from build123d import *

# Parameters (mm, degrees)
F1_DEPTH  = 15
F2_W      = 70
F2_H      = 100
F3_DEPTH  = 5
F4_W      = 40
F4_H      = 50
F5_DEPTH  = 25
F7_DEPTH  = 40
F9_DEPTH  = 40
F11_DEPTH = 3
F13_DEPTH = 1.5
F14_DEPTH = 1.5


with BuildPart() as f1:
    # F0 (on Front) → F1 (new body)
    with BuildSketch(Plane.XZ):
        with BuildLine():
            ThreePointArc((-80, 0), (-87.071068, -2.928932), (-90, -10))
            Line((-90, -10), (-90, -110))
            ThreePointArc((-90, -110), (-87.071068, -117.071068), (-80, -120))
            Line((-80, -120), (-10, -120))
            ThreePointArc((-10, -120), (-2.928932, -117.071068), (0, -110))
            Line((0, -110), (0, -10))
            ThreePointArc((0, -10), (-2.928932, -2.928932), (-10, 0))
            Line((-10, 0), (-80, 0))
        make_face()
    extrude(amount=F1_DEPTH)

    # F2 (on face) → F3 (cut)
    with BuildSketch(Plane.XZ.offset(15)):
        with Locations((-45, -60)):
            Rectangle(F2_W, F2_H)
    extrude(amount=-F3_DEPTH, mode=Mode.SUBTRACT)

    # F4 (on face) → F5 (join)
    with BuildSketch(Plane(origin=(0, 0, 0), x_dir=(-1, 0, 0), z_dir=(0, 1, 0))):
        with Locations((45, -25)):
            Rectangle(F4_W, F4_H)
    extrude(amount=F5_DEPTH)

    # F6 (on face) → F7 (cut)
    with BuildSketch(Plane(origin=(-65, 0, 0), x_dir=(0, -1, 0), z_dir=(-1, 0, 0))):
        Polygon((0, -39.708052), (0, 0), (-25, 0), align=None)
        Polygon((-25, -9.351011), (-25, -50), (0, -50), align=None)
    extrude(amount=-F7_DEPTH, mode=Mode.SUBTRACT)

    # F8 (on face) → F9 (cut)
    with BuildSketch(Plane(origin=(-65, 0, 0), x_dir=(0, -1, 0), z_dir=(-1, 0, 0))):
        with BuildLine():
            Line((-19.594347, -8.585918), (-25, 0))
            Line((-25, 0), (-25, -9.351011))
            Line((-25, -9.351011), (-24.627329, -8.520231))
            ThreePointArc((-24.627329, -8.520231), (-23.514035, -7.469649), (-21.983944, -7.513993))
            Line((-21.983944, -7.513993), (-19.594347, -8.585918))
        make_face()
    extrude(amount=-F9_DEPTH, mode=Mode.SUBTRACT)

    # F10 (on face) → F11 (join)
    with BuildSketch(Plane.XZ.offset(10)):
        Polygon((-20, -15), (-15, -20), (-15, -15), align=None)
        Polygon((-70, -105), (-75, -100), (-75, -105), align=None)
        Polygon((-75, -20), (-70, -15), (-75, -15), align=None)
        Polygon((-15, -100), (-20, -105), (-15, -105), align=None)
    extrude(amount=F11_DEPTH)

    # F12 (on face) → F13 (cut)
    with BuildSketch(Plane.XZ.offset(10)):
        Polygon((-74, -19), (-71, -16), (-74, -16), align=None)
        Polygon((-19, -16), (-16, -19), (-16, -16), align=None)
        Polygon((-71, -104), (-74, -101), (-74, -104), align=None)
        Polygon((-16, -101), (-19, -104), (-16, -104), align=None)
    extrude(amount=F13_DEPTH, mode=Mode.SUBTRACT)

    # F12 (on face) → F14 (cut)
    with BuildSketch(Plane.XZ.offset(10)):
        Polygon((-74, -19), (-71, -16), (-74, -16), align=None)
        Polygon((-19, -16), (-16, -19), (-16, -16), align=None)
        Polygon((-71, -104), (-74, -101), (-74, -104), align=None)
        Polygon((-16, -101), (-19, -104), (-16, -104), align=None)
    extrude(amount=F14_DEPTH, mode=Mode.SUBTRACT)


solid = f1.part
Work out the finished part from the listing and answer in its coordinate system (mm). A direction names the side the tool comes from. Coordinates: 2 decimals unless noted, no trailing zeros. Loops run counter-clockwise (first coordinate to the right, second up) from the corner with the lowest first, then second, coordinate; pieces in that order, holes last. Notation, with made-up numbers: (68.25, 35.25) -> (121.25, 35.25) arc R34 cw to (121.25, 74.25) -> close; hole circle Ø1 at (89, 14). An arc over 180 degrees is marked (long way). Write each question's results on one line, items separated by ' | '. Start each with the question number.
1) Consider line 1 along Z through (x, y) = (-26.5, -10.5); line 2 along X through (y, z) = (-12.5, -47); line 3 along Y through (x, z) = (-9, -56). Determine where each line is inside the solid, lowest interval first.
2) For faces 1 (the flat face through (-65, 11, -27)), 2 (the flat face through (-17, -11.5, -17)), 3 (the flat face through (-17, -12, -102)), 4 (the cylindrical face through (-86.99, -7.4, -2.85)), 5 (the cylindrical face through (-87.15, -7.4, -116.99)), determine the directions among +Z, -Z, +X, -X, +Y, -Y from which every point of the face is accessible in a straight line to the end or side of a thin tool.
3) Find section A-A on x = -23.5. Determine the outline of the cut face in (y, z).
4) The mould has two halves that part along Y. Classify faces 6 (the flat face through (-17, -11.5, -103)), 7 (the flat face through (-45.3, 12.3, -30)), 8 (the flat face through (-18, -12, -17)): pulls with the +Y half, pulls with the -Y half, needs draft (parallel to the pull), parting line crosses it, or undercut.
5) Find section C-C on z = -96.5. Determine the outline of the cut face in (x, y), then the cut area to 3 significant figures.
6) Find section D-D on x = -59. Determine the outline of the cut face in (y, z), then the cut area to 3 significant figures.
7) Flat-ended cylindrical pins translate along their axes: P1, Ø2.5, axis at x = -71.5, z = -16.5, coming from the -Y side; P2, Ø10, axis at x = -58.5, z = -60, coming from the +Y side; P3, Ø8, axis at x = -37.5, z = -50, coming from the -Y side; P4, Ø10, axis at y = 2.5, z = -19, coming from the -X side. Find the tip coordinate at first contact, or state that the pin passes through.
8) Find section B-B on z = -37.5. Determine the outline of the cut face in (x, y).
Response values:
1) line 1: z = -120 to -110, -10 to 0 | line 2: x = -90 to -80, -10 to 0 | line 3: y = -15 to 0
2) face 1: +Z, -Z, -X, +Y | face 2: none | face 3: -Y | face 4: +Z, -X, +Y, -Y | face 5: -Z, -X, +Y, -Y
3) outline: (-15, -120) -> (0, -120) -> (0, 0) -> (-15, 0) -> (-15, -10) -> (-10, -10) -> (-10, -110) -> (-15, -110) -> close
4) face 6: undercut | face 7: pulls with the +Y half | face 8: needs draft
5) outline: (-90, -15) -> (-80, -15) -> (-80, -10) -> (-10, -10) -> (-10, -15) -> (0, -15) -> (0, 0) -> (-90, 0) -> close | area: 1,000 mm^2
6) outline: (-15, -120) -> (0, -120) -> (0, -50) -> (25, -9.35) -> (24.63, -8.52) arc R2 ccw to (21.98, -7.51) -> (19.59, -8.59) -> (0, -39.71) -> (0, 0) -> (-15, 0) -> (-15, -10) -> (-10, -10) -> (-10, -110) -> (-15, -110) -> close | area: 1,530 mm^2
7) P1: stops at y = -13 | P2: stops at y = 0 | P3: stops at y = -10 | P4: stops at x = -90
8) outline: (-90, -15) -> (-80, -15) -> (-80, -10) -> (-10, -10) -> (-10, -15) -> (0, -15) -> (0, 0) -> (-90, 0) -> close; (-65, 1.39) -> (-25, 1.39) -> (-25, 7.69) -> (-65, 7.69) -> close
